Could you check a few things on this model? Use its own coordinates, in mm. A direction names the side the tool comes from. Coordinates: 2 decimals unless noted, no trailing zeros. Write each loop counter-clockwise with the first axis right and the second up, starting at its lowest first coordinate (ties: lowest second). Pieces come first, ordered by that corner, then holes. Notation, with made-up numbers: M -38.75,-30 L -29.75,-30 A12 ccw -29.75,-20 Z; hole C -7.75,65 d2. An arc over 180 degrees is marked long. Write item = value, one per line.
```python
from build123d import *

# Parameters (mm, degrees)
BOSS_EXTRUDE1_DEPTH = 59.69
SKETCH2_R           = 3.302
SKETCH2_R_2         = 1.397
CUT_EXTRUDE1_DEPTH  = 85.326589408
SKETCH3_R           = 3.175
CUT_EXTRUDE2_DEPTH  = 85.326589408
CUT_EXTRUDE3_DEPTH  = 2.06375


with BuildPart() as part:
    # Sketch1 → Boss-Extrude1 (new body)
    with BuildSketch(Plane(origin=(0, 0, 0), x_dir=(1, 0, 0), z_dir=(0, 1, 0))):
        Polygon((0, 0), (0, 20.447), (2.159, 20.447), (2.159, 14.2875), (6.223, 14.2875), (6.223, 58.4835), (11.303, 58.4835), (11.303, -5.0165), (6.223, -5.0165), (6.223, 6.1595), (2.159, 6.1595), (2.159, 0), align=None)
    extrude(amount=BOSS_EXTRUDE1_DEPTH)

    # Sketch2 → Cut-Extrude1 (cut, through all)
    with BuildSketch(Plane(origin=(11.303, 0, 0), x_dir=(0, 0, -1), z_dir=(1, 0, 0))):
        with Locations((43.561, 29.845)):
            Circle(SKETCH2_R)
        with Locations((43.561, 13.716)):
            Circle(SKETCH2_R_2)
        with Locations((43.561, 7.112)):
            Circle(SKETCH2_R_2)
        with Locations((43.561, 45.974)):
            Circle(SKETCH2_R_2)
        with Locations((43.561, 52.578)):
            Circle(SKETCH2_R_2)
    extrude(amount=-CUT_EXTRUDE1_DEPTH, mode=Mode.SUBTRACT)

    # Sketch3 → Cut-Extrude2 (cut, through all)
    with BuildSketch(Plane.ZY):
        with Locations((-10.2235, 48.26)):
            Circle(SKETCH3_R)
        with Locations((-10.2235, 11.43)):
            Circle(SKETCH3_R)
    extrude(amount=-CUT_EXTRUDE2_DEPTH, mode=Mode.SUBTRACT)

    # Sketch4 → Cut-Extrude3 (cut)
    with BuildSketch(Plane.ZY):
        Polygon((-14.7955, 8.790354569), (-14.7955, 14.069645431), (-10.2235, 16.709290861), (-5.6515, 14.069645431), (-5.6515, 8.790354569), (-10.2235, 6.150709139), align=None)
        Polygon((-14.7955, 45.620354569), (-14.7955, 50.899645431), (-10.2235, 53.539290861), (-5.6515, 50.899645431), (-5.6515, 45.620354569), (-10.2235, 42.980709139), align=None)
    extrude(amount=-CUT_EXTRUDE3_DEPTH, mode=Mode.SUBTRACT)


solid = part.part
```
Item 1: If we mould it in two halves opening along X, with no side actions, what happens to faces 4 (the face through (4, 29, -14.288)), 5 (the face through (0, 29, -10)), 6 (the face through (1.017, 7.452, -12.477))? For each: pulls with the +X half, pulls with the -X half, needs draft (parallel to the pull), parting line crosses it, or undercut.
Numbers:
face_4 = undercut
face_5 = pulls with the -X half
face_6 = needs draft
Item 2: For faces 1 (the face through (8.8, 12.35, -43.26)), 2 (the face through (2.159, 29, -3)), 3 (the face through (1.02, 15.37, -12.54)), which set-ups out of +Z, -Z, +X, -X, +Y, -Y let a thin tool reach every point of the face, with its end or its side?
Numbers:
face_1 = +X, -X
face_2 = +Z, +Y, -Y
face_3 = -X
Item 3: Imagine slicing it at A-A (y = 48.26). Write out the boundary of the cut face in (x, z), and give its area (3 significant figures).
Numbers:
outline = M 0,-20.45 L 2.16,-20.45 L 2.16,-14.29 L 6.22,-14.29 L 6.22,-58.48 L 11.3,-58.48 L 11.3,-13.4 L 2.06,-13.4 L 2.06,-14.8 L 0,-14.8 Z; M 0,-5.65 L 2.06,-5.65 L 2.06,-7.05 L 11.3,-7.05 L 11.3,5.02 L 6.22,5.02 L 6.22,-6.16 L 2.16,-6.16 L 2.16,0 L 0,0 Z
area = 322 mm²
Item 4: I'm going to push flat-ended pins straight in: P1, Ø0.6, axis at x = 0.5, y = 49, coming from the +Z side; P2, Ø1.7, axis at x = 1, y = 10.5, coming from the -Z side; P3, Ø3.5, axis at y = 13.716, z = -43.561, coming from the -X side; P4, Ø2, axis at y = 52.578, z = -43.561, coming from the +X side. Where does each tip first touch, or does it pass through?
Numbers:
P1 = 0
P2 = -20.45
P3 = 6.22
P4 = through
Item 5: Imagine slicing it at C-C (y = 36.5). Write out the boundary of the cut face in (x, z).
Numbers:
outline = M 0,-20.45 L 2.16,-20.45 L 2.16,-14.29 L 6.22,-14.29 L 6.22,-58.48 L 11.3,-58.48 L 11.3,5.02 L 6.22,5.02 L 6.22,-6.16 L 2.16,-6.16 L 2.16,0 L 0,0 Z
Item 6: Imagine slicing it at B-B (z = -18). Write out the boundary of the cut face in (x, y).
Numbers:
outline = M 0,0 L 2.16,0 L 2.16,59.69 L 0,59.69 Z; M 6.22,0 L 11.3,0 L 11.3,59.69 L 6.22,59.69 Z
Item 7: If I drill on line 1 along Y through (x, z) = (3, -12); line 2 along X through (y, z) = (36, -18.5); line 3 along Z through (x, y) = (1, 8.5), over which ranges is the centre line in solid material (lowest first)?
Numbers:
line_1 = 0 to 8.8, 14.06 to 45.63, 50.89 to 59.69
line_2 = 0 to 2.16, 6.22 to 11.3
line_3 = -20.45 to -14.29, -6.15 to 0
Item 8: Imagine slicing it at D-D (x = 4.5). State how many separate pieces and enclosed holes the cut face has, and give its area (3 significant figures).
Numbers:
separate_pieces = 1
enclosed_holes = 2
area = 422 mm²
